The figure shows three views and two pictorial views of one solid part (mm, origin at its lowest corner). Answer the questions. Coordinates: 2 decimals unless noted, no trailing zeros. Order: outer loops, then holes, each group sorted by start corner. A loop starts at its lowest first (then second) coordinate and runs counter-clockwise, first axis right, second up. Notation, with made-up numbers: (65.25, 82) - (74.25, 82) arc R13 ccw to (74.25, 97) - close; hole circle Ø9 at (52.25, 6.5). An arc over 180 degrees is marked (long way). Use one line per item in the form item = value.
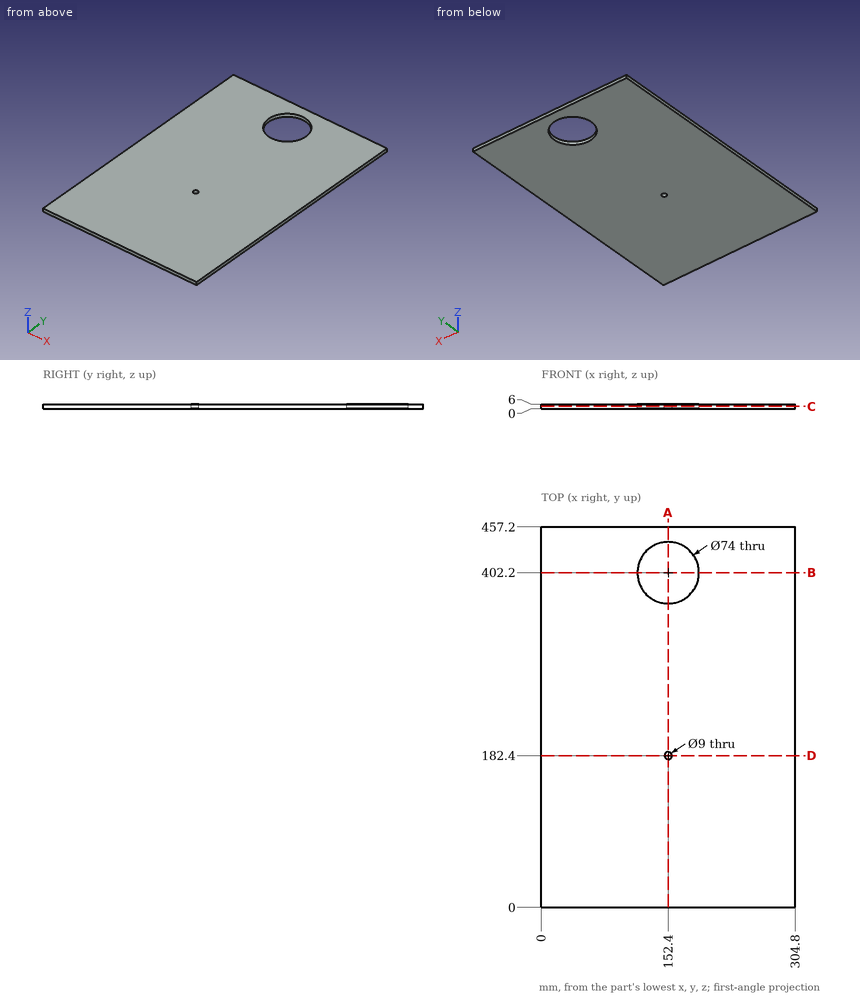
(1) Section B-B, the plane y = 402.2 is taken. Write down the section's boundary in (x, z), then the cut area to 3 significant figures.
Answer list:
outline = (0, 0) - (115.4, 0) - (115.4, 6) - (0, 6) - close; (189.4, 0) - (304.8, 0) - (304.8, 6) - (189.4, 6) - close
area = 1,380 mm2
(2) Given pin 1 Ø14.5 at (x, y) = (152.4, 182.4) entering from +Z, flat-ended and moving along its own axis, determine where the tip first touches the part or whether it passes through.
Answer list:
pin_1 = 6
(3) Section C-C, the plane z = 3.15 is taken. Write down the section's boundary in (x, y).
Answer list:
outline = (0, 0) - (304.8, 0) - (304.8, 457.2) - (0, 457.2) - close; hole circle Ø74 at (152.4, 402.2); hole circle Ø9 at (152.4, 182.4)
(4) Straight lines are drawn through the part: L1, parallel to Y at x = 152.4, z = 3.3; L2, parallel to X at y = 182.4, z = 3; L3, parallel to Y at x = 149, z = 3.4. For each, find the intervals that lie inside material, in ascending order.
Answer list:
L1 = 0 to 177.9, 186.9 to 365.2, 439.2 to 457.2
L2 = 0 to 147.9, 156.9 to 304.8
L3 = 0 to 179.45, 185.35 to 365.36, 439.04 to 457.2
(5) Section D-D, the plane y = 182.4 is taken. Write down the section's boundary in (x, z).
Answer list:
outline = (0, 0) - (147.9, 0) - (147.9, 6) - (0, 6) - close; (156.9, 0) - (304.8, 0) - (304.8, 6) - (156.9, 6) - close
(6) Section A-A, the plane x = 152.4 is taken. Write down the section's boundary in (y, z), then the cut area to 3 significant figures.
Answer list:
outline = (0, 0) - (177.9, 0) - (177.9, 6) - (0, 6) - close; (186.9, 0) - (365.2, 0) - (365.2, 6) - (186.9, 6) - close; (439.2, 0) - (457.2, 0) - (457.2, 6) - (439.2, 6) - close
area = 2,250 mm2
